CAD build for the part. Positions are in the model's coordinates, mm. Face numbers are marked on the shaded views. A direction names the side the tool comes from. Give positions to 0.01 mm unless a question says otherwise; leave off trailing zeros. Write each loop counter-clockwise with the first axis right and the second up, starting at its lowest first coordinate (ties: lowest second). Pieces come first, ordered by that corner, then holes. Notation, with made-up numbers: (2.25, -0.5) -> (15.25, -0.5) arc R21 cw to (15.25, 29.5) -> close; hole circle Ø5 at (-8, 71.5). An arc over 180 degrees is marked (long way). Answer as a JSON object with one key per item and string values.
```python
from build123d import *

# Parameters (mm, degrees)
BOSS_EXTRUDE1_DEPTH = 7.62


with BuildPart() as part:
    # Sketch1 → Boss-Extrude1 (new body)
    with BuildSketch(Plane(origin=(-22.749553377, 0, 0), x_dir=(0, 0, -1), z_dir=(1, 0, 0))):
        Polygon((-112.227241806, 51.836669294), (-105.877241806, 51.836669294), (-74.104597168, 36.364189717), (-42.072441806, 51.963044496), (-35.722441806, 51.963044496), (-35.722441806, 45.613044496), (-64.409753583, 31.643044496), (-35.722441806, 17.673044496), (-35.722441806, 11.323044496), (-42.072441806, 11.323044496), (-74.104597168, 26.921899275), (-105.877241806, 11.449419699), (-112.227241806, 11.449419699), (-112.227241806, 17.799419699), (-83.799440754, 31.643044496), (-112.227241806, 45.486669294), align=None)
    extrude(amount=-BOSS_EXTRUDE1_DEPTH)


solid = part.part
```
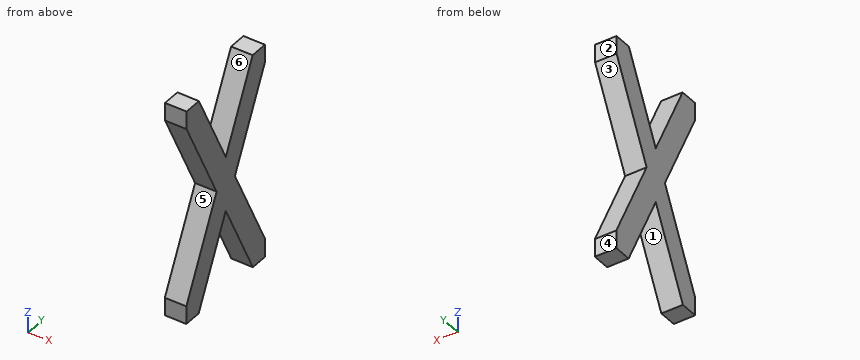
1) Slice it at B-B (x = -27). List the corners of the cut face in (y, z), then the cut area to 3 significant figures.
Model answer:
{"outline": "(11.32, 35.72) -> (17.67, 35.72) -> (31.64, 64.41) -> (45.61, 35.72) -> (51.96, 35.72) -> (51.96, 42.07) -> (36.36, 74.1) -> (51.84, 105.88) -> (51.84, 112.23) -> (45.49, 112.23) -> (31.64, 83.8) -> (17.8, 112.23) -> (11.45, 112.23) -> (11.45, 105.88) -> (26.92, 74.1) -> (11.32, 42.07) -> close", "area": "1,310 mm2"}
2) Mould opens along Y. For the marked faces 4, 5 and 6 say: released by +Y, released by -Y, zero draft, split by the parting line, or undercut.
Model answer:
{"face 4": "released by +Y", "face 5": "released by -Y", "face 6": "undercut"}
3) Slice it at C-C (z = 102). List the corners of the cut face in (x, y), then the cut area to 3 significant figures.
Model answer:
{"outline": "(-30.37, 13.34) -> (-22.75, 13.34) -> (-22.75, 22.78) -> (-30.37, 22.78) -> close; (-30.37, 40.51) -> (-22.75, 40.51) -> (-22.75, 49.95) -> (-30.37, 49.95) -> close", "area": "144 mm2"}
4) Wall check: probe 1 along Y at (x, z) = (-27.5, 102.5); probe 2 along Z at (x, y) = (-28.5, 44.5); probe 3 along Z at (x, y) = (-29.5, 47.5). Give the ranges that are in metal, low to high.
Model answer:
{"probe 1": "y = 13.09 to 22.54, 40.75 to 50.19", "probe 2": "z = 38.01 to 57.4, 90.81 to 110.2", "probe 3": "z = 35.72 to 51.24, 96.97 to 112.23"}
5) Slice it at A-A (y = 47.5). List the corners of the cut face in (x, z), then the cut area to 3 significant figures.
Model answer:
{"outline": "(-30.37, 35.72) -> (-22.75, 35.72) -> (-22.75, 51.24) -> (-30.37, 51.24) -> close; (-30.37, 96.97) -> (-22.75, 96.97) -> (-22.75, 112.23) -> (-30.37, 112.23) -> close", "area": "234 mm2"}
6) Slice it at D-D (z = 81). List the corners of the cut face in (x, y).
Model answer:
{"outline": "(-30.37, 23.56) -> (-22.75, 23.56) -> (-22.75, 39.72) -> (-30.37, 39.72) -> close"}
7) Pin check, flat tips, straight feed: pin 1 (1.5 mm diameter, centred on x = -25, y = 21.5, fed in from +Z); pin 2 (3 mm diameter, centred on x = -24.5, z = 80, fed in from +Y); pin 3 (1 mm diameter, centred on x = -29, z = 45.5, fed in from +Y). Stop position of each tip, or through.
Model answer:
{"pin 1": "stops at z = 106.17", "pin 2": "stops at y = 39.97", "pin 3": "stops at y = 50.54"}
8) 3-axis set-ups, long thin cutter, end or side, ignore diameter. For the marked faces 1, 2 and 3: which of +Z, -Z, +X, -X, +Y, -Y reach the whole face in a straight line?
Model answer:
{"face 1": "-Z, +X, -X", "face 2": "+Z, +X, -X, +Y", "face 3": "+X, -X, +Y"}
